```python
from build123d import *

# Parameters (mm, degrees)
PAD_DEPTH         = 2.5
SKETCH001_W       = 4
SKETCH001_H       = 2
POCKET_DEPTH      = 193.80181
POCKET_DEPTH_BACK = 193.80181
SKETCH002_W       = 4
SKETCH002_H       = 12
POCKET001_DEPTH   = 193.80181


with BuildPart() as part:
    # Sketch → Pad (new body, symmetric)
    with BuildSketch(Plane.XY):
        Polygon((-45, 0), (-15, 0), (-15, 12), (-45, 12), (-45, 22), (45, 22), (45, 12), (15, 12), (15, 0), (45, 0), (45, -10), (-45, -10), align=None)
    extrude(amount=PAD_DEPTH, both=True)

    # Sketch001 → Pocket (cut, two sides)
    with BuildSketch(Plane.XY) as pocket_sk:
        with Locations((-32, -3)):
            Rectangle(SKETCH001_W, SKETCH001_H)
        with Locations((-32, 15)):
            Rectangle(SKETCH001_W, SKETCH001_H)
        with Locations((-23, -3)):
            Rectangle(SKETCH001_W, SKETCH001_H)
        with Locations((-23, 15)):
            Rectangle(SKETCH001_W, SKETCH001_H)
    pocket = extrude(amount=-POCKET_DEPTH, mode=Mode.SUBTRACT) + extrude(pocket_sk.sketch, amount=POCKET_DEPTH_BACK, mode=Mode.SUBTRACT)

    # Mirrored: Pocket across YZ
    add(pocket.mirror(Plane.YZ), mode=Mode.SUBTRACT)

    # Sketch002 → Pocket001 (cut, through all)
    with BuildSketch(Plane.XY):
        with Locations((-7, -6)):
            Rectangle(SKETCH002_W, SKETCH002_H)
    pocket001 = extrude(amount=POCKET001_DEPTH, mode=Mode.SUBTRACT)

    # Mirrored001: Pocket001 across Sketch002 V_Axis
    add(pocket001.mirror(Plane(origin=(0, 0, 0), x_dir=(0, 0, 1), z_dir=(1, 0, 0))), mode=Mode.SUBTRACT)


solid = part.part
```
Here's how the part is built. I have some questions about the finished solid (model axes, mm). A direction names the side the tool comes from. Give positions to 0.01 mm unless a question says otherwise; leave off trailing zeros. Loops run counter-clockwise (first coordinate to the right, second up) from the corner with the lowest first, then second, coordinate; pieces in that order, holes last. Notation, with made-up numbers: M 47.5,8.25 L 78.5,8.25 A16 ccw 78.5,30.25 Z; hole C -22,-7.5 d1. An arc over 180 degrees is marked long. Return JSON: item names as keys, results as strings.
Item 1: Imagine slicing it at D-D on y = 7. List the corners of the cut face in (x, z) for me, then the cut area to 3 significant figures.
A:
{"outline": "M -15,-2.5 L 15,-2.5 L 15,2.5 L -15,2.5 Z", "area": "150 mm^2"}
Item 2: Thinking about a two-plate mould opening in X: for faces 4 (the flat face through (1, -10, 0)), 5 (the flat face through (-32, 16, 0)), 6 (the flat face through (-45, -5, 0)), which applies, released by +X, released by -X, zero draft, split by the parting line, or undercut?
A:
{"face 4": "zero draft", "face 5": "undercut", "face 6": "released by -X"}
Item 3: I'm going to push flat-ended pins straight in: pin 1 Ø2 at (y, z) = (1.5, 2) entering from -X; pin 2 Ø8 at (x, y) = (-31, 6.5) entering from +Z. Where does each tip first touch, or does it pass through?
A:
{"pin 1": "stops at x = -15", "pin 2": "passes through"}
Item 4: Please list where these lines run through material, in increasing order: line 1 (Y direction, x = 22, z = -0.3); line 2 (X direction, y = 15.5, z = 1.45); line 3 (Y direction, x = -38, z = 0.85).
A:
{"line 1": "y = -10 to -4, -2 to 0, 12 to 14, 16 to 22", "line 2": "x = -45 to -34, -30 to -25, -21 to 21, 25 to 30, 34 to 45", "line 3": "y = -10 to 0, 12 to 22"}
Item 5: On a 3-axis mill with a long thin cutter (end or side, diameter ignored), from which of +Z, -Z, +X, -X, +Y, -Y can I reach the whole of each face in a straight line? I mean faces 1 (the flat face through (23, 16, 0)), 2 (the flat face through (-15, 6, 0)), 3 (the flat face through (7, 0, 1)). Say none if no direction works.
A:
{"face 1": "+Z, -Z", "face 2": "+Z, -Z, -X", "face 3": "+Z, -Y"}
Item 6: Imagine slicing it at B-B on y = -7.5. List the corners of the cut face in (x, z) for me, then the cut area to 3 significant figures.
A:
{"outline": "M -45,-2.5 L 45,-2.5 L 45,2.5 L 9,2.5 L 9,0 L 5,0 L 5,2.5 L -5,2.5 L -5,0 L -9,0 L -9,2.5 L -45,2.5 Z", "area": "430 mm^2"}
Item 7: Imagine slicing it at A-A on x = -31. List the corners of the cut face in (y, z) for me.
A:
{"outline": "M -10,-2.5 L -4,-2.5 L -4,2.5 L -10,2.5 Z; M -2,-2.5 L 0,-2.5 L 0,2.5 L -2,2.5 Z; M 12,-2.5 L 14,-2.5 L 14,2.5 L 12,2.5 Z; M 16,-2.5 L 22,-2.5 L 22,2.5 L 16,2.5 Z"}
Item 8: Imagine slicing it at C-C on z = 1.65. State how many separate pieces and enclosed holes the cut face has, then the cut area to 3 significant figures.
A:
{"separate pieces": "1", "enclosed holes": "8", "area": "2,020 mm^2"}
